Input: dimensioned drawing with shaded views. Units: mm. Origin: part minimum x, y, z. A direction names the side the tool comes from. Round coordinates to 2 decimals unless told otherwise and drop trailing zeros. Loops run counter-clockwise (first coordinate to the right, second up) from the corner with the lowest first, then second, coordinate; pieces in that order, holes last. Notation, with made-up numbers: M 59,6.5 L 94,6.5 A31 ccw 94,31.5 Z; hole C -1.5,54.5 d8. An arc over 180 degrees is marked long. Use one line per item in the form item = value. Start each with the question number.
Q1. Mould query, pull axis Z, two halves, no side actions, for the marked faces 4, 5 and 6. Classes: pulls with the +Z half, pulls with the -Z half, needs draft (parallel to the pull), parting line crosses it, or undercut.
Q2. First-contact query: P1, Ø6, axis at x = 24, y = 21.5, coming from the -Z side; P2, Ø8, axis at x = 27.5, y = 20, coming from the +Z side; P3, Ø15, axis at x = 34, y = 14.5, coming from the -Z side; P4, Ø3, axis at y = 21.5, z = 6.5, coming from the -X side. Flat tips, straight axial feed; report the tip coordinate or a pass-through.
Q3. Section query B-B, the plane z = 81. Output: boundary loops of the cut face in (x, y), and give its area (3 significant figures).
Q4. Section query C-C, the plane x = 27.5. Output: boundary loops of the cut face in (y, z), and give its area (3 significant figures).
Q5. Section query D-D, the plane y = 3.25. Output: boundary loops of the cut face in (x, z).
Q6. Section query A-A, the plane y = 17. Output: boundary loops of the cut face in (x, z).
Q7. Ray query, line 1 along Y through (x, z) = (27, 98); line 2 along X through (y, z) = (18.75, 70.5); line 3 along Z through (x, y) = (9, 14). Return the intervals inside material, ascending.
Q8. Access query for the marked faces 1, 2 and 3. Directions: +Z, -Z, +X, -X, +Y, -Y. A direction counts if a zero-diameter tool reaches every point of the face in a straight line with its end or side. Return the directions, or none.
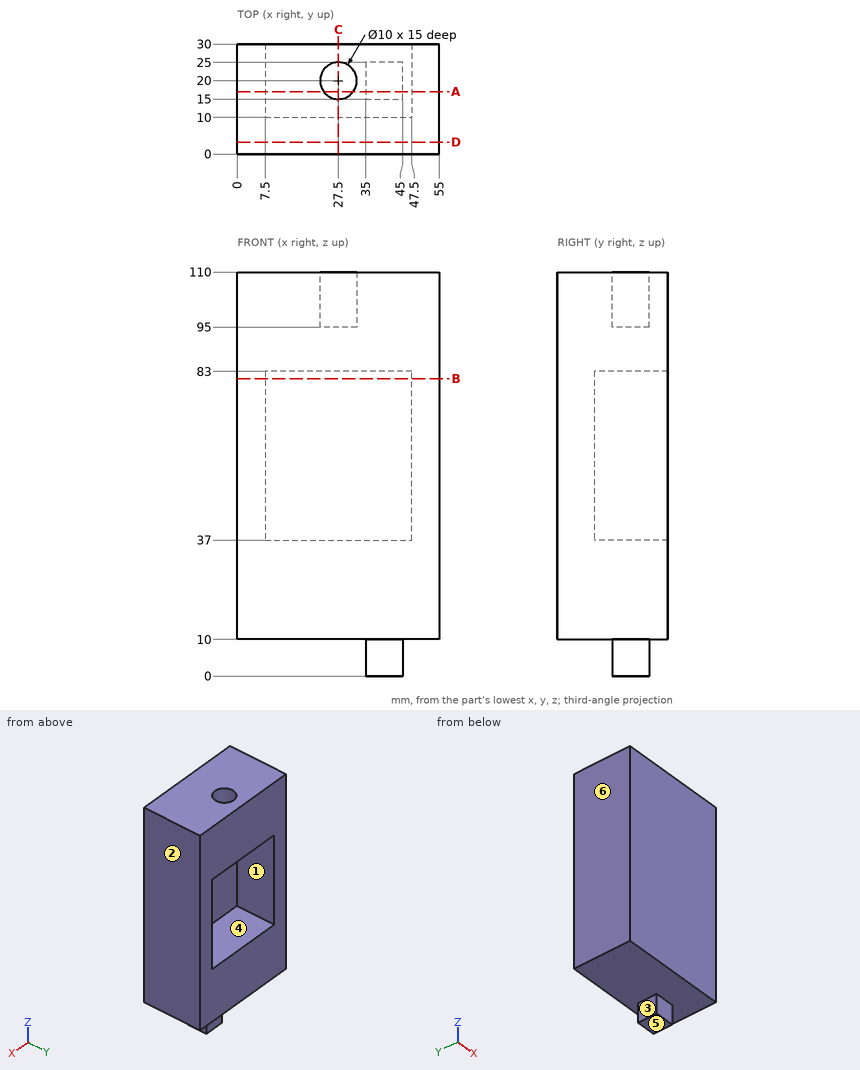
Results found:
q1.face_4 = undercut
q1.face_5 = pulls with the -Z half
q1.face_6 = needs draft
q2.P1 = 10
q2.P2 = 95
q2.P3 = 0
q2.P4 = 35
q3.outline = M 0,0 L 55,0 L 55,30 L 47.5,30 L 47.5,10 L 7.5,10 L 7.5,30 L 0,30 Z
q3.area = 850 mm²
q4.outline = M 0,10 L 30,10 L 30,37 L 10,37 L 10,83 L 30,83 L 30,110 L 25,110 L 25,95 L 15,95 L 15,110 L 0,110 Z
q4.area = 1,930 mm²
q5.outline = M 0,10 L 55,10 L 55,110 L 0,110 Z
q6.outline = M 0,10 L 35,10 L 35,0 L 45,0 L 45,10 L 55,10 L 55,110 L 31.5,110 L 31.5,95 L 23.5,95 L 23.5,110 L 0,110 Z; hole M 7.5,37 L 47.5,37 L 47.5,83 L 7.5,83 Z
q7.line_1 = 0 to 15.03, 24.97 to 30
q7.line_2 = 0 to 7.5, 47.5 to 55
q7.line_3 = 10 to 37, 83 to 110
q8.face_1 = +Y
q8.face_2 = +Z, -Z, +X, +Y, -Y
q8.face_3 = -Z, -X, +Y, -Y
